Autodesk Inventor part; units mm, degrees
ref_plane "YZ Plane" through (0, 0, 0) normal (1, 0, 0) x (0, 1, 0)
ref_plane "XZ Plane" through (0, 0, 0) normal (0, 1, 0) x (-1, 0, 0)
ref_plane "XY Plane" through (0, 0, 0) normal (0, 0, 1) x (1, 0, 0)
sketch "Sketch1" plane through (0, 0, 0) normal (0, 0, 1) x (1, 0, 0)
  line L0 (0, 0) -> (72, 0)
  line L1 (72, 0) -> (72, 130)
  line L2 (72, 130) -> (0, 130)
  line L3 (0, 130) -> (0, 0)
  dimension "d0" = 72
  dimension "d1" = 130
extrude "Extrusion1" add sketch "Sketch1" against normal blind 5
fillet "Fillet1" radius 4 1 edges at (72, 130, -2.5)
fillet "Fillet2" radius 4 1 edges at (0, 130, -2.5)
sketch "Sketch2" plane through (0, 0, -5) normal (0, 0, -1) x (-1, 0, 0)
  circle A0 centre (-67, 125) radius 1.5
  line L0 (-72, 126) -> (-72, 0)
  line L1 (-4, 130) -> (-68, 130)
  line L2 (0, 0) -> (0, 126)
  arc A1 (0, 126) -> (-4, 130) centre (-4, 126) ccw
  line L3 (-4, 130) -> (-68, 130)
  arc A2 (-68, 130) -> (-72, 126) centre (-68, 126) ccw
  line L4 (-72, 126) -> (-72, 0)
  line L5 (-72, 0) -> (0, 0)
  line L6 (0, 0) -> (0, 126)
  line L7 (-68, 130) -> (-4, 130)
  line L8 (0, 0) -> (-72, 0)
  circle A3 centre (-5, 125) radius 1.5
  circle A4 centre (-67, 5) radius 1.5
  line L9 (-36, 130) -> (-36, 0)
  circle A5 centre (-5, 5) radius 1.5
  dimension "d7" = 3
  dimension "d8" = 5
  dimension "d9" = 5
  dimension "d10" = 3
  dimension "d11" = 5
  dimension "d12" = 5
hole "Hole1" at (67, 125, -5) at (5, 125, -5) at (67, 5, -5) at (5, 5, -5) direction (0, 0, 1) diameter 2.6416 depth 10.979
properties part number "backdor" material "Steel"
Geometry check sheet. Reference: the model listing, model coordinates, mm. Coordinates: 2 decimals unless noted, no trailing zeros. Loops run counter-clockwise (first coordinate to the right, second up) from the corner with the lowest first, then second, coordinate; pieces in that order, holes last. Notation, with made-up numbers: (-25.5, 72.25) - (3.5, 72.25) arc R10 ccw to (3.5, 79.25) - close; hole circle Ø3 at (-9.75, 20.25). An arc over 180 degrees is marked (long way). One line per item, written item: value. Start each with the question number.
(1) Cross-section at A-A on y = 5. Enter the section's corners in (x, z).
(2) Material ranges on line 1 (Y direction, x = 5, z = -3); line 2 (X direction, y = 5, z = -3), recorded low to high. Write a range as [from, to].
(3) Mould release check, pull along X, two halves, no side actions. Record for faces 1 (the cylindrical face through (65.69, 4.83, -2.46)), 2 (the flat face through (35, 66, 0)), 3 (the flat face through (72, 62, -2)): released by +X, released by -X, zero draft, split by the parting line, or undercut.
Results below:
1. outline: (0, -5) - (3.68, -5) - (3.68, 0) - (0, 0) - close; (6.32, -5) - (65.68, -5) - (65.68, 0) - (6.32, 0) - close; (68.32, -5) - (72, -5) - (72, 0) - (68.32, 0) - close
2. line 1: y = [0, 3.68], [6.32, 123.68], [126.32, 130]
2. line 2: x = [0, 3.68], [6.32, 65.68], [68.32, 72]
3. face 1: undercut
3. face 2: zero draft
3. face 3: released by +X
